For this review, take the finished solid that the model builds, in its own axes (mm). Face numbers are marked on the shaded views. A direction names the side the tool comes from. Round coordinates to 2 decimals unless told otherwise and drop trailing zeros. Write each loop counter-clockwise with the first axis right and the second up, starting at its lowest first coordinate (ties: lowest second). Pieces come first, ordered by that corner, then holes. Notation, with made-up numbers: (2, 3.5) -> (13, 3.5) arc R19 ccw to (13, 17.5) -> close; hole circle Ø11 at (-9, 79). An arc over 180 degrees is marked (long way). Answer in a Markdown table with one row per item. Add a question column.
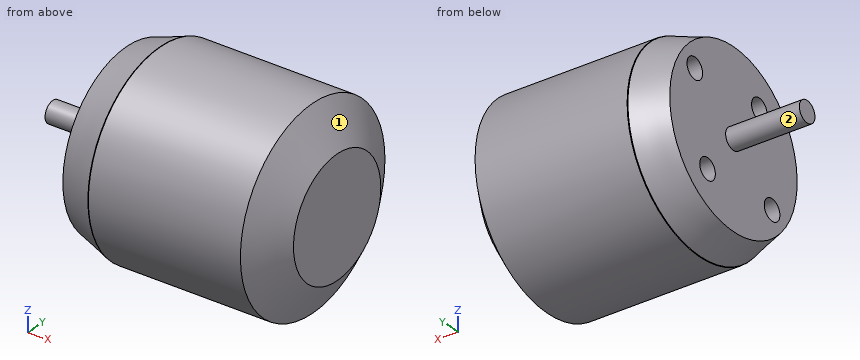
```python
from build123d import *

# Parameters (mm, degrees)
SKETCH2_R          = 1.5
CUT_EXTRUDE1_DEPTH = 10


with BuildPart() as part:
    # Sketch1 → Revolve2 (revolve)
    with BuildSketch(Plane.XY, mode=Mode.PRIVATE) as revolve2_sk:
        Polygon((-25.236130379, 13.869097433), (-30, 12.25), (-30, 1.5), (-40.5, 1.5), (-40.5, 0), (0, 0), (0, 8.396394587), (-3.485025076, 13.9), (-25.145205772, 13.9), (-25.145205772, 6.9), (-25.236130379, 6.858374097), align=None)
    revolve(revolve2_sk.sketch.rotate(Axis((-72.504474406, 0, 0), (1, 0, 0)), 90), axis=Axis((-72.504474406, 0, 0), (1, 0, 0)))

    # Sketch2 → Cut-Extrude1 (cut)
    with BuildSketch(Plane.ZY.offset(30)):
        with Locations((5.918430072, 7.431163131)):
            Circle(SKETCH2_R)
        with Locations((-6.257821584, 4.983941113)):
            Circle(SKETCH2_R)
        with Locations(Location((6.257821584, -4.983941113, 0), (0, 0, 180))):
            Circle(SKETCH2_R)
        with Locations((-5.918430072, -7.431163131)):
            Circle(SKETCH2_R)
    extrude(amount=-CUT_EXTRUDE1_DEPTH, mode=Mode.SUBTRACT)


solid = part.part
```
1. We need section B-B (x = -19). Write out the cut boundary in (y, z), plus the area to 3 significant figures.
2. Tool access review of the marked faces 1 and 2: name each direction out of +Z, -Z, +X, -X, +Y, -Y from which nothing blocks a thin tool from reaching the whole face with its end or side.
3. We need section D-D (x = -27). Write out the cut boundary in (y, z), plus the area to 3 significant figures.
4. Clearance check with flat-ended pins moving along their axes: pin 1 Ø2 at (x, z) = (-28, 5) entering from +Y; pin 2 Ø8 at (x, y) = (-21.5, 10.5) entering from -Z; pin 3 Ø3.5 at (y, z) = (8, 6.5) entering from -X; pin 4 Ø1 at (x, z) = (-33.5, 2.5) entering from +Y. State where each tip first meets the part, or that it passes through.
5. We need section A-A (z = 0). Write out the cut boundary in (x, y), plus the area to 3 significant figures.
6. For L1, parallel to X at y = -1.5, z = 2.5; L2, parallel to Y at x = -17, z = 0; L3, parallel to Y at x = -5, z = -3, list the stretches that pass through material, from the lowest coordinate up. Write a range as [from, to].
Response:
| question | item | result |
|---|---|---|
| 1 | outline | circle Ø27.8 at (0, 0) |
| 1 | area | 607 mm2 |
| 2 | face 1 | +X |
| 2 | face 2 | -X |
| 3 | outline | circle Ø26.54 at (0, 0); hole circle Ø3 at (-7.43, -5.92); hole circle Ø3 at (-4.98, 6.26); hole circle Ø3 at (4.98, -6.26); hole circle Ø3 at (7.43, 5.92) |
| 3 | area | 525 mm2 |
| 4 | pin 1 | y = 12.45 |
| 4 | pin 2 | z = -12.29 |
| 4 | pin 3 | x = -30 |
| 4 | pin 4 | through |
| 5 | outline | (-40.5, -1.5) -> (-30, -1.5) -> (-30, -12.25) -> (-25.24, -13.87) -> (-25.24, -6.86) -> (-25.15, -6.9) -> (-25.15, -13.9) -> (-3.49, -13.9) -> (0, -8.4) -> (0, 8.4) -> (-3.49, 13.9) -> (-25.15, 13.9) -> (-25.15, 6.9) -> (-25.24, 6.86) -> (-25.24, 13.87) -> (-30, 12.25) -> (-30, 1.5) -> (-40.5, 1.5) -> close |
| 5 | area | 837 mm2 |
| 6 | L1 | [-30, 0] |
| 6 | L2 | [-13.9, 13.9] |
| 6 | L3 | [-13.57, 13.57] |
